Autodesk Inventor part; units mm, degrees
ref_plane "YZ Plane" through (0, 0, 0) normal (1, 0, 0) x (0, 1, 0)
ref_plane "XZ Plane" through (0, 0, 0) normal (0, 1, 0) x (-1, 0, 0)
ref_plane "XY Plane" through (0, 0, 0) normal (0, 0, 1) x (1, 0, 0)
sketch "Sketch1" plane through (0, 0, 0) normal (0, 0, 1) x (1, 0, 0)
  line L0 (0, 25.4) -> (0, 0)
  line L1 (0, 0) -> (25.4, 0)
  line L2 (3.175, 25.4) -> (3.175, 4.953)
  line L3 (4.953, 3.175) -> (25.4, 3.175)
  line L4 (0, 25.4) -> (3.175, 25.4)
  line L5 (25.4, 3.175) -> (25.4, 0)
  line L6 (3.175, 4.953) -> (3.175, 3.175)
  line L7 (4.953, 3.175) -> (3.175, 3.175)
  dimension "d0" = 25.4
  dimension "d1" = 25.4
  dimension "d2" = 3.175
extrude "Extrusion1" add sketch "Sketch1" along normal blind 492.125
sketch "Sketch7" plane through (3.175, 3.175, 0) normal (1, 0, 0) x (0, 0, -1)
  circle A0 centre (-479.425, 9.525) radius 2.8124
  line L0 (0, 22.225) -> (-492.125, 22.225)
  line L1 (-492.125, 0) -> (-492.125, 22.225)
  circle A1 centre (-12.7, 9.525) radius 2.8124
  point P0 (0, -3.175)
  dimension "d43" = 12.7
  dimension "d44" = 12.7
  dimension "d47" = 466.725
hole "mount" at (3.175, 12.7, 479.425) at (3.175, 12.7, 12.7) direction (-1, 0, 0) diameter 6.7564 depth 25.4 tip angle 118
sketch "Sketch8" plane through (3.175, 3.175, 0) normal (0, 1, 0) x (1, 0, 0)
  line L0 (-3.175, -492.125) -> (22.225, -492.125)
  line L1 (9.525, -492.125) -> (9.525, 0) construction
  line L2 (22.225, 0) -> (22.225, -492.125)
  circle A0 centre (9.525, -246.0625) radius 4.5971
  point P0 (-3.175, 0)
  dimension "d59" = 12.7
hole "Hole5" at (12.7, 3.175, 246.0625) direction (0, -1, 0) diameter 6.7564 depth 25.4 tip angle 118
properties part number "angle_L104"
Geometry: final body of the model. Coordinates: model frame, mm. A direction names the side the tool comes from. Round coordinates to 2 decimals unless told otherwise and drop trailing zeros. Order: outer loops, then holes, each group sorted by start corner. A loop starts at its lowest first (then second) coordinate and runs counter-clockwise, first axis right, second up. Notation, with made-up numbers: M 30,-30.5 L 70,-30.5 A15 cw 70,-25.5 Z; hole C 86,4.5 d9. An arc over 180 degrees is marked long. One line per item, written item: value.
(1) Line query: probe 1 along Z at (x, y) = (0.8, 12.7) (3 decimals); probe 2 along Z at (x, y) = (12.7, 1.8) (3 decimals); probe 3 along X at (y, z) = (8.5, 318.5) (3 decimals). Output: solid intervals per line, ascending. Write a range as [from, to].
Result sheet:
probe 1: [0, 9.322], [16.078, 476.047], [482.803, 492.125]
probe 2: [0, 242.684], [249.441, 492.125]
probe 3: [0, 3.175]
(2) Cut plane A-A (z = 123). Return the cut outline in (x, y) (3 decimals), and give its area (3 significant figures).
Result sheet:
outline: M 0,0 L 25.4,0 L 25.4,3.175 L 3.175,3.175 L 3.175,25.4 L 0,25.4 Z
area: 151 mm2
(3) Cut plane B-B (x = 21). Return the cut outline in (y, z) (3 decimals), and give its area (3 significant figures).
Result sheet:
outline: M 0,0 L 3.175,0 L 3.175,492.125 L 0,492.125 Z
area: 1,560 mm2
(4) Reachability of faces 1 (the flat face through (3.175, 14, 243)), 2 (the flat face through (15, 0, 243)) from +Z, -Z, +X, -X, +Y, -Y: full face, straight path, thin tool, end or side. Return the list, or none.
Result sheet:
face 1: +Z, -Z, +X, +Y
face 2: +Z, -Z, +X, -X, -Y
(5) Pin query (flat end, axial travel): P1, Ø5.5, axis at y = 12.7, z = 479.425, coming from the -X side; P2, Ø1.5, axis at x = 15.5, z = 337, coming from the +Y side (3 decimals); P3, Ø5, axis at y = 21, z = 257.5, coming from the +X side (3 decimals). Return the tip coordinate at first contact, or that it passes through.
Result sheet:
P1: through
P2: y = 3.175
P3: x = 3.175
